Autodesk Inventor part; units mm, degrees
ref_plane "YZ Plane" through (0, 0, 0) normal (1, 0, 0) x (0, 1, 0)
ref_plane "XZ Plane" through (0, 0, 0) normal (0, 1, 0) x (-1, 0, 0)
ref_plane "XY Plane" through (0, 0, 0) normal (0, 0, 1) x (1, 0, 0)
sketch "Sketch1" plane through (0, 0, 0) normal (0, 1, 0) x (-1, 0, 0)
  line L0 (0, -55.88) -> (-12.7, -55.88)
  line L1 (-12.7, 0) -> (0, 0)
  line L2 (0, 0) -> (0, -20.94)
  line L3 (0, -34.94) -> (0, -55.88)
  line L4 (-12.7, -55.88) -> (-12.7, -34.94)
  line L5 (-12.7, -20.94) -> (-12.7, 0)
  line L6 (0, -20.94) -> (0, -34.94)
  line L7 (-12.7, -20.94) -> (-12.7, -34.94)
  dimension "d1" = 55.88
  dimension "d2" = 12.7
extrude "Extrusion1" add sketch "Sketch1" along normal blind 1.5
sketch "Sketch2" plane through (0, 1.5, 0) normal (0, 1, 0) x (1, 0, 0)
  line L0 (12.7, 0) -> (12.7, 55.88)
  line L1 (12.7, 0) -> (10.16, 0)
  line L2 (12.7, 2.54) -> (12.7, 0)
  circle A0 centre (10.16, 2.54) radius 1.092
  circle A1 centre (10.16, 53.34) radius 1.092
  point P0 (0, 0)
  dimension "d8" = 2.184
  dimension "d10" = 2.184
extrude "Extrusion2" cut sketch "Sketch2" against normal blind 1.5
sketch "Sketch5" plane through (0, 0, 0) normal (0, 0, 1) x (1, 0, 0)
  line L0 (12.7, 0) -> (0, 0)
  line L1 (6.35, 0) -> (6.35, 1.5)
  line L2 (12.7, 1.5) -> (0, 1.5)
  line L3 (0, 0) -> (0, 1.5)
  line L4 (0, 0.75) -> (12.7, 0.75)
  line L5 (12.7, 0) -> (12.7, 1.5)
  circle A0 centre (6.35, 0.75) radius 5.175
  dimension "d30" = 10.35
extrude "Extrusion5" add sketch "Sketch5" along normal blind 1 contours A0 L0 | L0 L1 L4 A0 | L0 A0 L4 L1 | L4 L1 L2 A0 | L4 A0 L2 L1 | L2 A0
sketch "Sketch6" plane through (6.35, 0.75, 1) normal (0, 0, 1) x (1, 0, 0)
  circle A0 centre (0, 0) radius 5.175
  circle A1 centre (0, 0) radius 3.175
  point P0 (-6.35, -0.75)
  dimension "d35" = 6.35
extrude "Extrusion6" add sketch "Sketch6" along normal blind 9
sketch "Sketch7" plane through (12.7, 0, -55.88) normal (0, 0, -1) x (-1, 0, 0)
  line L0 (0, 0) -> (0, 1.5)
  line L1 (0, 0.75) -> (12.7, 0.75)
  line L2 (12.7, 0) -> (12.7, 1.5)
  line L3 (11.4704, 1.5) -> (1.2296, 1.5)
  line L4 (6.35, 1.5) -> (6.35, 0)
  circle A0 centre (6.35, 0.75) radius 5.175
extrude "Extrusion7" add sketch "Sketch7" along normal blind 1
sketch "Sketch8" plane through (6.35, 0.75, -56.88) normal (0, 0, -1) x (-1, 0, 0)
  circle A0 centre (0, 0) radius 5.175
  circle A1 centre (0, 0) radius 3.175
  point P0 (6.35, -0.75)
  dimension "d40" = 6.35
extrude "Extrusion8" add sketch "Sketch8" along normal blind 9
thread "Thread1"
thread "Thread2"
sketch "Sketch9" plane through (0, 0, 0) normal (0, 0, -1) x (-1, 0, 0)
  arc A0 (-11.4704, 0) -> (-1.2296, 0) centre (-6.35, 0.75) ccw
  line L0 (0, 0) -> (-1.2296, 0)
  line L1 (-11.4704, 0) -> (-1.2296, 0)
  circle A1 centre (-6.35, 0.75) radius 5.175
extrude "Extrusion9" add sketch "Sketch9" along normal up to next contours L1 A0
sketch "Sketch10" plane through (10.16, 0, -2.54) normal (0, 1, 0) x (1, 0, 0)
  circle A0 centre (0, 0) radius 1.092
  circle A1 centre (0, 50.8) radius 1.092
  circle A2 centre (0, 50.8) radius 1.092
  point P0 (-10.16, -2.54)
  dimension "d60" = 2.184
extrude "Extrusion10" cut sketch "Sketch10" against normal up to next
sketch "Sketch12" plane through (0, 1.5, 0) normal (0, 1, 0) x (1, 0, 0)
  circle A0 centre (10.16, 2.54) radius 1.092
  circle A1 centre (10.16, 2.54) radius 1.092
  circle A2 centre (10.16, 2.54) radius 2.2225
  circle A3 centre (10.16, 53.34) radius 1.092
  circle A4 centre (10.16, 53.34) radius 1.092
  circle A5 centre (10.16, 53.34) radius 2.2225
  point P0 (0, 0)
  dimension "d54" = 4.445
  dimension "d55" = 4.445
extrude "Extrusion11" cut sketch "Sketch12" against normal blind 5.925
sketch "Sketch13" plane through (0, 1.5, 0) normal (0, 1, 0) x (1, 0, 0)
  line L0 (12.7, 0) -> (12.7, 55.88)
  line L1 (12.7, 55.88) -> (0, 55.88)
  line L2 (0, 55.88) -> (0, 0)
  line L3 (0, 0) -> (12.7, 0)
  line L4 (12.7, 0) -> (12.7, 55.88)
  circle A0 centre (10.16, 53.34) radius 1.092
  circle A1 centre (10.16, 53.34) radius 1.092
  circle A2 centre (10.16, 2.54) radius 1.092
  circle A3 centre (10.16, 2.54) radius 1.092
extrude "Extrusion12" add sketch "Sketch13" along normal blind 10.4775
thread "Thread5"
thread "Thread6"
sketch "Sketch14" plane through (10.16, 1.5, -53.34) normal (0, -1, 0) x (1, 0, 0)
  circle A0 centre (0, 0) radius 1.092
  circle A1 centre (0, 0) radius 2.2225
  circle A2 centre (0, 50.8) radius 2.2225
  circle A3 centre (0, 50.8) radius 2.2225
  circle A4 centre (0, 0) radius 1.092
  circle A5 centre (0, 50.8) radius 1.092
  point P0 (-10.16, 53.34)
extrude "Extrusion13" cut sketch "Sketch14" against normal blind 1
sketch "Sketch15" plane through (0, 11.9775, 0) normal (0, 1, 0) x (1, 0, 0)
  line L0 (12.7, 0) -> (12.7, 6.985)
  line L1 (12.7, 0) -> (12.7, 55.88)
  line L2 (12.7, 0) -> (19.685, 0) construction
  line L3 (11.525, -10) -> (11.525, 65.88)
  line L4 (11.43, 6.985) -> (13.97, 6.985) construction
  line L5 (11.43, 6.985) -> (12.43, 6.985) construction
  line L6 (11.43, 9.525) -> (12.43, 9.525) construction
  line L7 (12.7, 5.985) -> (12.7, 10.525)
  line L8 (12.7, 5.985) -> (12.7, 5.485)
  line L9 (12.7, 5.485) -> (9.93, 5.485)
  line L10 (9.93, 5.485) -> (9.93, 11.025)
  line L11 (9.93, 11.025) -> (12.7, 11.025)
  line L12 (12.7, 11.025) -> (12.7, 10.525)
  point P0 (0, 0)
  dimension "d72" = 90
  dimension "d130" = 0.5
  dimension "d131" = 2.77
  dimension "d132" = 5.54
extrude "Extrusion14" cut sketch "Sketch15" against normal blind 8
sketch "Sketch16" plane through (0, 11.9775, 0) normal (0, 1, 0) x (1, 0, 0)
  line L0 (12.7, 0) -> (12.7, 55.88)
  line L1 (12.7, 40.234) -> (13.97, 40.234) construction
  line L2 (0, 0) -> (12.7, 0)
  line L3 (11.43, 0) -> (40.005, 0) construction
  line L4 (11.525, -10) -> (11.525, 65.88)
  line L5 (11.43, 28.575) -> (13.97, 28.575) construction
  line L6 (11.43, 46.355) -> (12.43, 46.355) construction
  line L7 (11.43, 28.575) -> (13.97, 28.575) construction
  line L8 (11.43, 20.955) -> (12.43, 20.955) construction
  line L9 (6.89, 19.955) -> (6.89, 47.355)
  line L10 (12.7, 47.355) -> (12.7, 19.955)
  line L11 (6.89, 47.355) -> (6.89, 47.855)
  line L12 (6.89, 47.855) -> (12.7, 47.855)
  line L13 (12.7, 47.855) -> (12.7, 47.355)
  line L14 (12.7, 19.955) -> (12.7, 19.455)
  line L15 (12.7, 0) -> (12.7, 55.88)
  line L16 (12.7, 19.455) -> (6.89, 19.455)
  line L17 (6.89, 19.455) -> (6.89, 19.955)
  point P0 (12.7, 10.525)
  dimension "d123" = 5.81
  dimension "d129" = 28.4
extrude "Extrusion15" cut sketch "Sketch16" against normal blind 8 contours L16 L4 L12 L0 | L16 L17 L9 L11 L12 L4
properties part number "Line Sensor 6 Bracket 2.0"
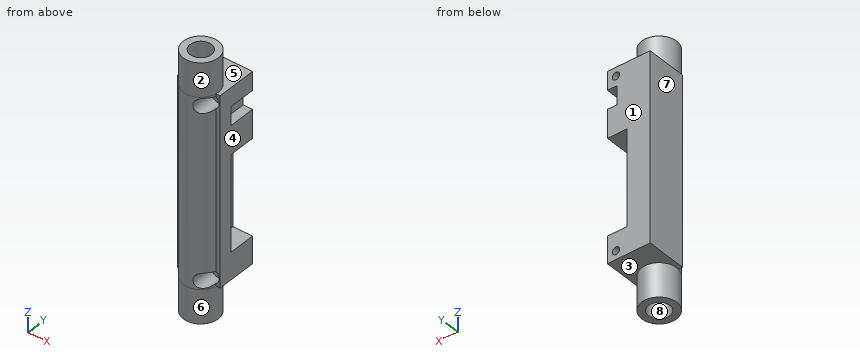
For this review, take the finished solid that the model builds, in its own axes (mm). Face numbers are marked on the shaded views. A direction names the side the tool comes from. Round coordinates to 2 decimals unless told otherwise and drop trailing zeros. Write each loop counter-clockwise with the first axis right and the second up, starting at its lowest first coordinate (ties: lowest second). Pieces come first, ordered by that corner, then holes. Notation, with made-up numbers: M 83.5,42 L 95.5,42 A22 ccw 95.5,53 Z; hole C -35.75,83.5 d7. An arc over 180 degrees is marked long. One line per item, written item: value. Start each with the question number.
(1) Machinability: for the marked faces 1, 2, 3, 4 and 5, which of the approach directions +Z, -Z, +X, -X, +Y, -Y give a long, thin tool a straight path to every point of the face, cutting with its end or side? Answer none if there is none.
(2) We need section A-A (z = -53.34). Give the boundary of the cut face in (x, y).
(3) We need section D-D (y = 5.25). Give the boundary of the cut face in (x, z) (1 decimal), and give its area (3 significant figures).
(4) We need section C-C (z = -13). Give the boundary of the cut face in (x, y).
(5) Wall thickness on line 1 (Z direction, x = 10.16, y = 0); line 2 (Z direction, x = 10.16, y = 8) (3 decimals); line 3 (Z direction, x = 12, y = 11) (3 decimals): over which ranges is each line inside the solid? List them lowest first.
(6) We need section B-B (y = 0.75). Give the boundary of the cut face in (x, z) (1 decimal).
(7) The part is to be moulded in two halves that separate along X. For the marked faces 6, 7 and 8, say which applies: released by +X, released by -X, zero draft, split by the parting line, or undercut.
(8) Insertion check: pin 1 (4 mm diameter, centred on x = 6.35, y = 0.75, fed in from -Z); pin 2 (1.4 mm diameter, centred on x = 11.5, y = 7.5, fed in from +Z); pin 3 (3 mm diameter, centred on x = 4, z = -58, fed in from -Y). Each pin has a flat end and moves straight along its axis. Give the tip position at first contact, or say it passes through.
Result:
1. face 1: +Z, -Z, +X, -X, +Y
1. face 2: +Z
1. face 3: -Z, +Y
1. face 4: +Z, -Z, +X, +Y, -Y
1. face 5: +Z, +Y
2. outline: M 0,0 L 1.23,0 A5.18 ccw 7.94,-4.18 L 7.94,2.5 L 9.07,2.5 L 9.07,11.98 L 0,11.98 Z; M 11.25,2.5 L 12.38,2.5 L 12.38,0 L 12.7,0 L 12.7,11.98 L 11.25,11.98 Z
3. outline: M 0,-55.9 L 3.8,-55.9 L 3.8,-65.9 L 8.9,-65.9 L 8.9,-55.9 L 12.7,-55.9 L 12.7,-47.9 L 6.9,-47.9 L 6.9,-19.5 L 12.7,-19.5 L 12.7,-11 L 9.9,-11 L 9.9,-5.5 L 12.7,-5.5 L 12.7,0 L 8.9,0 L 8.9,10 L 3.8,10 L 3.8,0 L 0,0 Z; hole C 10.2,-53.3 d2.2; hole C 10.2,-2.5 d2.2
3. area: 624 mm²
4. outline: M 0,0 L 1.23,0 A5.18 ccw 11.47,0 L 12.7,0 L 12.7,11.98 L 0,11.98 Z
5. line 1: -65.88 to -55.56, -51.12 to -4.76, -0.32 to 10
5. line 2: -55.88 to -54.432, -52.248 to -47.855, -19.455 to -11.025, -5.485 to -3.632, -1.448 to 0
5. line 3: -55.88 to -47.855, -19.455 to -11.025, -5.485 to 0
6. outline: M 0,-55.9 L 1.2,-55.9 L 1.2,-65.9 L 3.2,-65.9 L 3.2,-56.9 L 9.5,-56.9 L 9.5,-65.9 L 11.5,-65.9 L 11.5,-55.9 L 12.7,-55.9 L 12.7,0 L 11.5,0 L 11.5,10 L 9.5,10 L 9.5,1 L 3.2,1 L 3.2,10 L 1.2,10 L 1.2,0 L 0,0 Z; hole C 10.2,-53.3 d4.4; hole C 10.2,-2.5 d4.4
7. face 6: split by the parting line
7. face 7: released by -X
7. face 8: undercut
8. pin 1: z = -56.88
8. pin 2: z = 0
8. pin 3: y = -4.35
